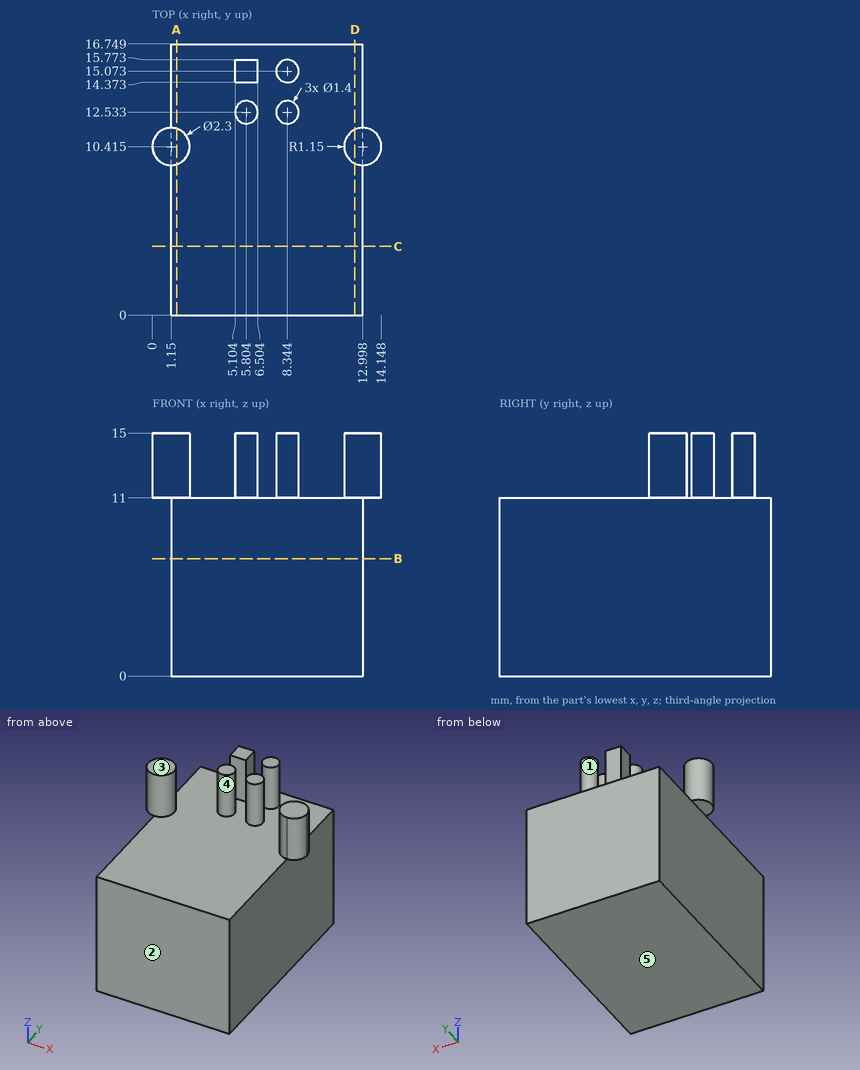
The figure shows three views and two pictorial views of one solid part (mm, origin at its lowest corner). Answer the questions. A direction names the side the tool comes from. Round coordinates to 2 decimals unless told otherwise and drop trailing zeros. Write each loop counter-clockwise with the first axis right and the second up, starting at its lowest first coordinate (ties: lowest second). Pieces come first, ordered by that corner, then holes. Notation, with made-up numbers: (84, 31.25) -> (127, 31.25) arc R12 ccw to (127, 50.25) -> close; hole circle Ø9 at (35, 37). An arc over 180 degrees is marked (long way). Answer as a JSON object with one key per item and string values. Group by question number.
Q1. Each of these flat-tipped pins is pushed along its axis until it touches: pin 1 Ø3.5 at (y, z) = (7, 3) entering from +X; pin 2 Ø0.7 at (y, z) = (15, 13) entering from -X; pin 3 Ø1.1 at (y, z) = (14.5, 13.5) entering from +X. Where does it stop, or does it pass through?
Q2. Section D-D (x = 12.5) is taken. Write down the section's boundary in (y, z).
Q3. Section C-C (y = 4.25) is taken. Write down the section's boundary in (x, z).
Q4. Section A-A (x = 1.5) is taken. Write down the section's boundary in (y, z).
Q5. Straight lines are drawn through the part: line 1 along Z through (x, y) = (6.25, 5.75); line 2 along X through (y, z) = (5, 1); line 3 along Y through (x, z) = (13, 13.5) (1 decimal). For each, find the intervals that lie inside material, in ascending order.
Q6. Section B-B (z = 7.25) is taken. Write down the section's boundary in (x, y).
Q7. Determine the mould class of the marked faces 1, 2 and 3 for opening direction Y: pulls with the +Y half, pulls with the -Y half, needs draft (parallel to the pull), parting line crosses it, or undercut.
Q8. Which of the six approach directions +Z, -Z, +X, -X, +Y, -Y give full straight-line access (tool end or side, diameter ignored) to the marked faces 4 and 5?
Check values:
{
 "1": {"pin 1": "x = 13", "pin 2": "x = 5.1", "pin 3": "x = 9.04"},
 "2": {"outline": "(0, 0) -> (16.75, 0) -> (16.75, 11) -> (11.45, 11) -> (11.45, 15) -> (9.38, 15) -> (9.38, 11) -> (0, 11) -> close"},
 "3": {"outline": "(1.15, 0) -> (13, 0) -> (13, 11) -> (1.15, 11) -> close"},
 "4": {"outline": "(0, 0) -> (16.75, 0) -> (16.75, 11) -> (11.51, 11) -> (11.51, 15) -> (9.32, 15) -> (9.32, 11) -> (0, 11) -> close"},
 "5": {"line 1": "0 to 11", "line 2": "1.15 to 13", "line 3": "9.3 to 11.6"},
 "6": {"outline": "(1.15, 0) -> (13, 0) -> (13, 16.75) -> (1.15, 16.75) -> close"},
 "7": {"face 1": "undercut", "face 2": "pulls with the -Y half", "face 3": "needs draft"},
 "8": {"face 4": "+Z", "face 5": "-Z, +X, -X, +Y, -Y"}
}
